Here's how the part is built. I have some questions about the finished solid (model axes, mm). Face numbers are marked on the shaded views. A direction names the side the tool comes from. Give positions to 0.01 mm unless a question says otherwise; leave off trailing zeros. Write each loop counter-clockwise with the first axis right and the second up, starting at its lowest first coordinate (ties: lowest second). Pieces come first, ordered by that corner, then holes. Notation, with made-up numbers: (-31, 27) -> (4, 27) arc R12 ccw to (4, 32) -> close; hole circle Ø1 at (-24, -35). An arc over 180 degrees is marked (long way). Return JSON: item names as keys, results as strings.
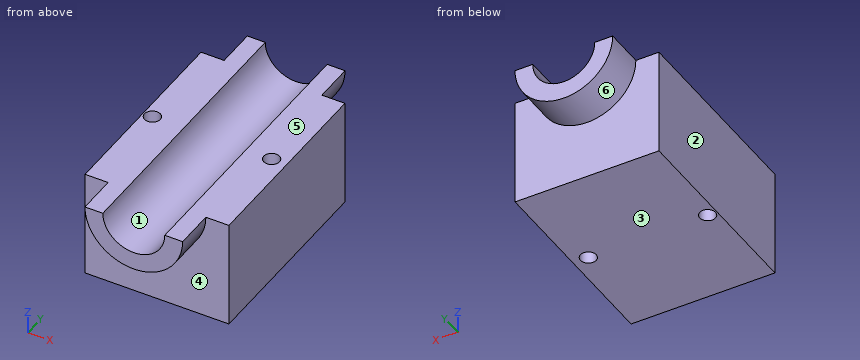
from build123d import *

# Parameters (mm, degrees)
F0_W     = 91.506348
F0_H     = 68.513646
F1_DEPTH = 63.5
F3_DEPTH = 25.4
F5_DEPTH = 152.401
F7_DEPTH = 25.4
F8_R     = 5.041929
F9_DEPTH = 68.514647


with BuildPart() as f1:
    # F0 (on Front) → F1 (new body, symmetric)
    with BuildSketch(Plane.XZ):
        Rectangle(F0_W, F0_H)
    extrude(amount=F1_DEPTH, both=True)

    # F2 (on face) → F3 (join)
    with BuildSketch(Plane.XZ.offset(63.5)):
        with BuildLine():
            Line((-19.708274, 34.256823), (-31.091106, 34.256823))
            ThreePointArc((-31.091106, 34.256823), (0, 3.165717), (31.091106, 34.256823))
            Line((31.091106, 34.256823), (19.708274, 34.256823))
            ThreePointArc((19.708274, 34.256823), (0, 14.548549), (-19.708274, 34.256823))
        make_face()
    extrude(amount=F3_DEPTH)

    # F4 (on face) → F5 (cut, through all)
    with BuildSketch(Plane.XZ.offset(88.9)):
        with BuildLine():
            Line((19.708274, 34.256823), (-19.708274, 34.256823))
            ThreePointArc((-19.708274, 34.256823), (0, 14.548549), (19.708274, 34.256823))
        make_face()
    extrude(amount=-F5_DEPTH, mode=Mode.SUBTRACT)

    # F6 (on face) → F7 (join)
    with BuildSketch(Plane(origin=(0, 63.5, 0), x_dir=(-1, 0, 0), z_dir=(0, 1, 0))):
        with BuildLine():
            ThreePointArc((-31.091106, 34.256823), (0, 3.165717), (31.091106, 34.256823))
            Line((31.091106, 34.256823), (19.708274, 34.256823))
            ThreePointArc((19.708274, 34.256823), (0, 14.548549), (-19.708274, 34.256823))
            Line((-19.708274, 34.256823), (-31.091106, 34.256823))
        make_face()
    extrude(amount=F7_DEPTH)

    # F8 (on face) → F9 (cut, through all)
    with BuildSketch(Plane.XY.offset(34.256823)):
        with Locations((36.037404, 0)):
            Circle(F8_R)
        with Locations((-39.830811, 0)):
            Circle(F8_R)
    extrude(amount=-F9_DEPTH, mode=Mode.SUBTRACT)


solid = f1.part
1. For pin 1 Ø6 at (x, z) = (12, -9.5) entering from +Y; pin 2 Ø13 at (x, y) = (36.04, 0) entering from +Z; pin 3 Ø5 at (x, y) = (12.5, 46.5) entering from +Z; pin 4 Ø1.5 at (x, y) = (-8.5, 36) entering from +Z, each with a flat end and sliding along its axis, tell me the tip position at first contact or that it passes through.
Taken from the geometry:
{"pin 1": "stops at y = 63.5", "pin 2": "stops at z = 34.26", "pin 3": "stops at z = 21.47", "pin 4": "stops at z = 16.85"}
2. Suppose I cut it at C-C, the plane x = 0. List the corners of the cut face in (y, z) for me.
Taken from the geometry:
{"outline": "(-88.9, 3.17) -> (-63.5, 3.17) -> (-63.5, -34.26) -> (63.5, -34.26) -> (63.5, 3.17) -> (88.9, 3.17) -> (88.9, 14.55) -> (-88.9, 14.55) -> close"}
3. If we mould it in two halves opening along X, with no side actions, what happens to the marked faces 1, 2 and 3? For each: released by +X, released by -X, zero draft, split by the parting line, or undercut.
Taken from the geometry:
{"face 1": "undercut", "face 2": "released by -X", "face 3": "zero draft"}
4. If I drill on line 1 (X direction, y = -2, z = -28.5); line 2 (Y direction, x = -33, z = 10); line 3 (X direction, y = -64.5, z = 21.5), over which ranges is the centre line in solid material (lowest first)? Write a range as [from, to].
Taken from the geometry:
{"line 1": "x = [-45.75, -44.46], [-35.2, 31.41], [40.67, 45.75]", "line 2": "y = [-63.5, 63.5]", "line 3": "x = [-28.35, -15.02], [15.02, 28.35]"}
5. Suppose I cut it at D-D, the plane x = -22.5. List the corners of the cut face in (y, z) for me.
Taken from the geometry:
{"outline": "(-88.9, 12.8) -> (-63.5, 12.8) -> (-63.5, -34.26) -> (63.5, -34.26) -> (63.5, 12.8) -> (88.9, 12.8) -> (88.9, 34.26) -> (-88.9, 34.26) -> close"}
6. Suppose I cut it at B-B, the plane z = -9.5. List the corners of the cut face in (x, y) for me, and give its area (3 significant figures).
Taken from the geometry:
{"outline": "(-45.75, -63.5) -> (45.75, -63.5) -> (45.75, 63.5) -> (-45.75, 63.5) -> close; hole circle Ø10.08 at (-39.83, 0); hole circle Ø10.08 at (36.04, 0)", "area": "11,500 mm²"}
7. Which directions (+Z, -Z, +X, -X, +Y, -Y) give clear straight access to the entire face, cutting with the end or side of a thin tool? Please do the marked faces 4, 5 and 6.
Taken from the geometry:
{"face 4": "-Z, -Y", "face 5": "+Z, +X, -X, +Y, -Y", "face 6": "-Z, +Y"}
8. Suppose I cut it at A-A, the plane y = 0. List the corners of the cut face in (x, z) for me, and give its area (3 significant figures).
Taken from the geometry:
{"outline": "(-45.75, -34.26) -> (-44.87, -34.26) -> (-44.87, 34.26) -> (-45.75, 34.26) -> close; (-34.79, -34.26) -> (31, -34.26) -> (31, 34.26) -> (19.71, 34.26) arc R19.71 cw to (-19.71, 34.26) -> (-34.79, 34.26) -> close; (41.08, -34.26) -> (45.75, -34.26) -> (45.75, 34.26) -> (41.08, 34.26) -> close", "area": "4,280 mm²"}
